Could you check a few things on this drawing? It's one solid part, dimensions in mm from its lowest x, y, z. Coordinates: 2 decimals unless noted, no trailing zeros. Order: outer loops, then holes, each group sorted by start corner. A loop starts at its lowest first (then second) coordinate and runs counter-clockwise, first axis right, second up.
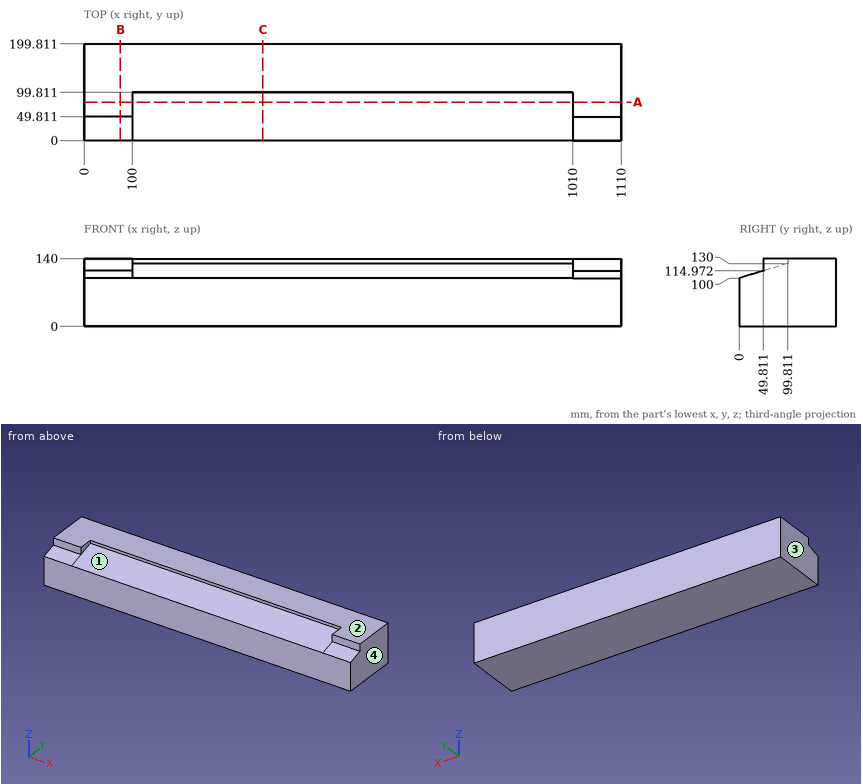
1. Please list where these lines run through material, in increasing order: probe 1 along Y at (x, z) = (63, 126.5); probe 2 along Z at (x, y) = (192, 68); probe 3 along Z at (x, y) = (537, 22.5).
Completed:
probe 1: y = 49.81 to 199.81
probe 2: z = 0 to 120.44
probe 3: z = 0 to 106.76
2. I'm going to push flat-ended pins straight in: pin 1 (2 mm diameter, centred on x = 231.5, y = 167, fed in from -Z); pin 2 (6 mm diameter, centred on x = 481.5, y = 35.5, fed in from +Z). Where does each tip first touch, or does it pass through?
Completed:
pin 1: stops at z = 0
pin 2: stops at z = 111.57
3. Thinking about a two-plate mould opening in X: for the marked faces 1, 2, 3 and 4, which applies, pulls with the +X half, pulls with the -X half, needs draft (parallel to the pull), parting line crosses it, or undercut?
Completed:
face 1: undercut
face 2: needs draft
face 3: pulls with the -X half
face 4: pulls with the +X half
4. Imagine slicing it at A-A on y = 79.5. Please give me the cut outline in (x, z) (1 decimal), then the cut area to 3 significant figures.
Completed:
outline: (0, 0) - (1110, 0) - (1110, 140) - (1010, 140) - (1010, 123.9) - (100, 123.9) - (100, 140) - (0, 140) - close
area: 141,000 mm2
5. Imagine slicing it at C-C on x = 369.5. Please give me the cut outline in (y, z).
Completed:
outline: (0, 0) - (199.81, 0) - (199.81, 140) - (99.81, 140) - (99.81, 130) - (0, 100) - close
6. Imagine slicing it at B-B on x = 75. Please give me the cut outline in (y, z), then the cut area to 3 significant figures.
Completed:
outline: (0, 0) - (199.81, 0) - (199.81, 140) - (49.81, 140) - (49.81, 114.97) - (0, 100) - close
area: 26,400 mm2
